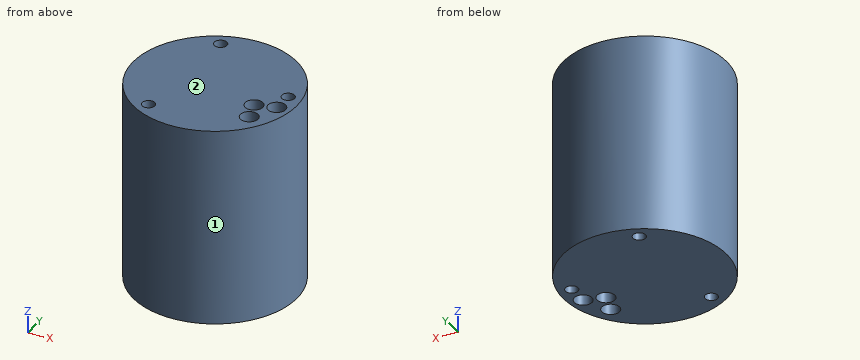
Autodesk Inventor part; units mm, degrees
ref_plane "YZ Plane" through (0, 0, 0) normal (1, 0, 0) x (0, 1, 0)
ref_plane "XZ Plane" through (0, 0, 0) normal (0, 1, 0) x (-1, 0, 0)
ref_plane "XY Plane" through (0, 0, 0) normal (0, 0, 1) x (1, 0, 0)
sketch "Sketch1" plane through (0, 0, 0) normal (0, 0, 1) x (1, 0, 0)
  circle A0 centre (0, 0) radius 11.5
  dimension "d0" = 23
extrude "Extrusion1" add sketch "Sketch1" along normal blind 28
sketch "Sketch2" plane through (0, 0, 28) normal (0, 0, 1) x (1, 0, 0)
  circle A0 centre (0, 0) radius 11.5
  line L0 (0, -16.1) -> (0, 16.1)
  line L1 (-16.1, 0) -> (16.1, 0)
  point P0 (0, 9.69)
  point P1 (-8.3918, -4.845)
  point P2 (8.3918, -4.845)
  point P3 (-4.074, 8.737)
  point P4 (-4.82, -8.349)
  point P5 (9.494, 1.674)
  dimension "d3" = 9.69
  dimension "d6" = 360
  dimension "d8" = 8.737
  dimension "d9" = 4.074
  dimension "d10" = 4.82
  dimension "d11" = 8.349
  dimension "d12" = 9.494
  dimension "d13" = 1.674
hole "Hole1" at (-4.074, 8.737, 28) at (-4.82, -8.349, 28) at (9.494, 1.674, 28) direction (0, 0, -1) diameter 1.778 end through all
sketch "Sketch3" plane through (0, 0, 28) normal (0, 0, 1) x (1, 0, 0)
  circle A0 centre (9.494, 1.674) radius 0.889
  circle A1 centre (-4.82, -8.349) radius 0.889
  circle A2 centre (-4.074, 8.737) radius 0.889
  circle A3 centre (0, 0) radius 11.5
  circle A4 centre (0, 0) radius 11.5
  point P0 (0, 9.69)
  point P1 (-8.3918, -4.845)
  point P2 (8.3918, -4.845)
  point P3 (4.074, -8.737)
  point P4 (4.82, 8.349)
  point P5 (-9.494, -1.674)
  dimension "d23" = 360
  dimension "d24" = -8.737
  dimension "d25" = 8.349
  dimension "d26" = 1.674
  dimension "d27" = 4.074
  dimension "d28" = 4.82
sketch "Sketch4" plane through (0, 0, 28) normal (0, 0, 1) x (1, 0, 0)
  point P0 (9.494, -1.2485)
  point P1 (6.7309, -2.117)
  point P2 (7.5994, -4.8853)
hole "Hole2" at (9.494, -1.2485, 28) at (6.7309, -2.117, 28) at (7.5994, -4.8853, 28) direction (0, 0, -1) diameter 2.5 end through all
properties part number "Connector_PCB"
Work out the finished part from the listing and answer in its coordinate system (mm). Face numbers are marked on the shaded views. Coordinates: 2 decimals unless noted, no trailing zeros. Loops run counter-clockwise (first coordinate to the right, second up) from the corner with the lowest first, then second, coordinate; pieces in that order, holes last. Notation, with made-up numbers: (59, 34) - (109, 34) arc R17 cw to (109, 56) - close; hole circle Ø6 at (8, 89). An arc over 180 degrees is marked (long way). Use a Markdown table: item, result.
Item 1: Consider probe 1 along X at (y, z) = (-1.75, 19.75); probe 2 along Y at (x, z) = (9.25, 7.25); probe 3 along X at (y, z) = (-1.5, 20.75). Determine where each line is inside the solid, lowest interval first. Write a range as from..to.
Evaluation:
| item | result |
|---|---|
| probe 1 | x = -11.37..5.54, 7.93..8.35, 10.64..11.37 |
| probe 2 | y = -6.83..-2.47, -0.02..0.82, 2.53..6.83 |
| probe 3 | x = -11.4..5.64, 7.82..8.27, 10.72..11.4 |
Item 2: The mould has two halves that part along X. Classify the marked faces 1 and 2: +X half, -X half, draft (parallel to the pull), parting line (faces both ways), or undercut.
Evaluation:
| item | result |
|---|---|
| face 1 | parting line |
| face 2 | draft |
Item 3: Find section C-C, the plane z = 2.25. State how many separate pieces and enclosed holes the cut face has, and give its area (3 significant figures).
Evaluation:
| item | result |
|---|---|
| separate pieces | 1 |
| enclosed holes | 6 |
| area | 393 mm2 |
Item 4: Find section B-B, the plane y = -2. Determine the outline of the cut face in (x, z).
Evaluation:
| item | result |
|---|---|
| outline | (-11.32, 0) - (5.49, 0) - (5.49, 28) - (-11.32, 28) - close; (7.98, 0) - (8.5, 0) - (8.5, 28) - (7.98, 28) - close; (10.49, 0) - (11.32, 0) - (11.32, 28) - (10.49, 28) - close |
Item 5: Given pin 1 Ø6 at (y, z) = (6.5, 7) entering from -X; pin 2 Ø3 at (x, z) = (-5, 19.5) entering from +Y; pin 3 Ø4 at (x, z) = (8.5, 19.5) entering from +Y, each flat-ended and moving along its own axis, determine where each tip first touches the part or whether it passes through.
Evaluation:
| item | result |
|---|---|
| pin 1 | stops at x = -10.95 |
| pin 2 | stops at y = 10.95 |
| pin 3 | stops at y = 9.49 |
Item 6: Find section D-D, the plane y = 5.25. Determine the outline of the cut face in (x, z).
Evaluation:
| item | result |
|---|---|
| outline | (-10.23, 0) - (10.23, 0) - (10.23, 28) - (-10.23, 28) - close |
Item 7: Find section A-A, the plane x = 7.25. Determine the outline of the cut face in (y, z).
Evaluation:
| item | result |
|---|---|
| outline | (-8.93, 0) - (-6.09, 0) - (-6.09, 28) - (-8.93, 28) - close; (-3.69, 0) - (-3.25, 0) - (-3.25, 28) - (-3.69, 28) - close; (-0.98, 0) - (8.93, 0) - (8.93, 28) - (-0.98, 28) - close |
